The model under review builds one solid part; all positions refer to its coordinate system, in mm. Face numbers are marked on the shaded views. A direction names the side the tool comes from. Give positions to 0.01 mm unless a question says otherwise; leave off trailing zeros. Loops run counter-clockwise (first coordinate to the right, second up) from the corner with the lowest first, then second, coordinate; pieces in that order, holes last. Notation, with made-up numbers: M 74.5,44 L 91.5,44 A19 ccw 91.5,74 Z; hole C 11.25,-9.75 d4. An arc over 180 degrees is marked long. Write item = value, one per line. Start each with the question number.
1. We need section B-B on y = -20. Give the boundary of the cut face in (x, z).
2. We need section C-C on x = -39.5. Give the boundary of the cut face in (y, z), then the cut area to 3 significant figures.
3. For the marked faces 1 and 2, list the 3-axis set-ups (+Z, -Z, +X, -X, +Y, -Y) from which the entire face can be reached by the end or side of a thin tool; tool diameter is ignored.
4. We need section A-A on z = 81. Give the boundary of the cut face in (x, y), then the cut area to 3 significant figures.
5. For pin 1 (7 mm diameter, centred on y = -10, z = 243, fed in from -X); pin 2 (1.5 mm diameter, centred on x = -32.5, z = 37.5, fed in from +Y); pin 3 (4 mm diameter, centred on x = -25.5, y = -8, fed in from -Z), all flat-tipped, find the tip position at first contact; note any pin that passes through.
6. Wall thickness on line 1 along X through (y, z) = (-2.5, 328); line 2 along Y through (x, z) = (-29.5, 332.5): over which ranges is each line inside the solid? List them lowest first. Write a range as from..to.
from build123d import *

# Parameters (mm, degrees)
SKETCH1_W           = 25.4
SKETCH1_H           = 25.4
BOSS_EXTRUDE1_DEPTH = 355.6
SKETCH3_W           = 26.173809645
SKETCH3_H           = 26.478044322
CUT_EXTRUDE2_DEPTH  = 355.6
SKETCH5_R           = 3.556
CUT_EXTRUDE3_DEPTH  = 358.409680899


with BuildPart() as part:
    # Sketch1 → Boss-Extrude1 (new body)
    with BuildSketch(Plane.XY):
        with Locations((-35.089575682, -12.7)):
            Rectangle(SKETCH1_W, SKETCH1_H)
    extrude(amount=BOSS_EXTRUDE1_DEPTH)

    # Sketch3 → Cut-Extrude2 (cut)
    with BuildSketch(Plane.XY.offset(355.6)):
        with Locations((-37.127480504, -10.509977839)):
            Rectangle(SKETCH3_W, SKETCH3_H)
    extrude(amount=-CUT_EXTRUDE2_DEPTH, mode=Mode.SUBTRACT)

    # Sketch5 → Cut-Extrude3 (cut, through all)
    with BuildSketch(Plane(origin=(-22.389575682, 0, 0), x_dir=(0, 0, -1), z_dir=(1, 0, 0))):
        with Locations(Location((-18.288, -11.648501303, 0), (0, 0, 90))):
            Circle(SKETCH5_R)
    extrude(amount=-CUT_EXTRUDE3_DEPTH, mode=Mode.SUBTRACT)


solid = part.part
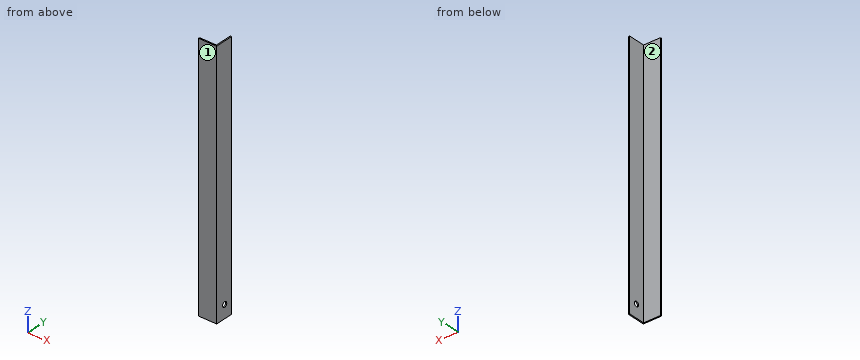
Final values:
q1.outline = M -24.04,0 L -22.39,0 L -22.39,355.6 L -24.04,355.6 Z
q2.outline = M -25.4,0 L -23.75,0 L -23.75,355.6 L -25.4,355.6 Z
q2.area = 587 mm²
q3.face_1 = +Z, -Z, +X, -X, -Y
q3.face_2 = +Z, -Z, -X, +Y
q4.outline = M -47.79,-25.4 L -22.39,-25.4 L -22.39,0 L -24.04,0 L -24.04,-23.75 L -47.79,-23.75 Z
q4.area = 81.1 mm²
q5.pin_1 = -24.04
q5.pin_2 = -23.75
q5.pin_3 = 0
q6.line_1 = -24.04..-22.39
q6.line_2 = -25.4..-23.75
